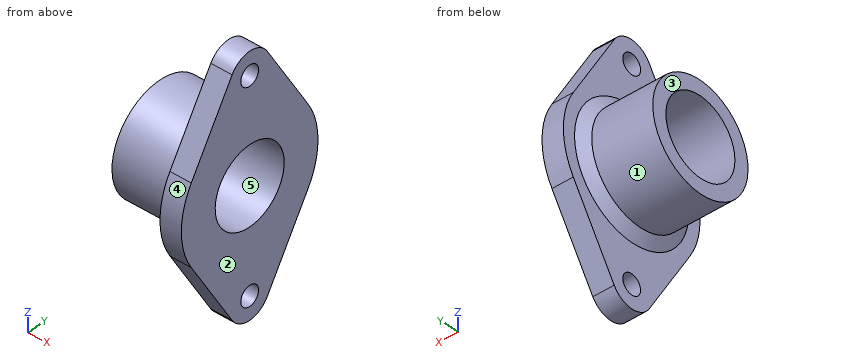
from build123d import *

# Parameters (mm, degrees)
BOSS_EXTRUDE1_DEPTH = 14
SKETCH2_R           = 6.5
CUT_EXTRUDE1_DEPTH  = 98.479485021
SKETCH3_R           = 25.25
CUT_EXTRUDE2_DEPTH  = 98.479485021
BOSS_EXTRUDE2_START = 45
SKETCH4_R           = 34.85
SKETCH4_R_2         = 25.25
BOSS_EXTRUDE2_DEPTH = 45


with BuildPart() as part:
    # Sketch1 → Boss-Extrude1 (new body)
    with BuildSketch(Plane(origin=(0, 0, 0), x_dir=(0, 0, -1), z_dir=(1, 0, 0))):
        with BuildLine():
            Line((-25.925925926, 42.753319928), (-75.277777778, 12.825995978))
            ThreePointArc((-75.277777778, 12.825995978), (-82.5, 0), (-75.277777778, -12.825995978))
            Line((-75.277777778, -12.825995978), (-25.925925926, -42.753319928))
            ThreePointArc((-25.925925926, -42.753319928), (0, -50), (25.925925926, -42.753319928))
            Line((25.925925926, -42.753319928), (75.277777778, -12.825995978))
            ThreePointArc((75.277777778, -12.825995978), (82.5, 0), (75.277777778, 12.825995978))
            Line((75.277777778, 12.825995978), (25.925925926, 42.753319928))
            ThreePointArc((25.925925926, 42.753319928), (0, 50), (-25.925925926, 42.753319928))
        make_face()
    extrude(amount=BOSS_EXTRUDE1_DEPTH)

    # Sketch2 → Cut-Extrude1 (cut, through all)
    with BuildSketch(Plane.ZY):
        with Locations((67.5, 0)):
            Circle(SKETCH2_R)
        with Locations((-67.5, 0)):
            Circle(SKETCH2_R)
    extrude(amount=-CUT_EXTRUDE1_DEPTH, mode=Mode.SUBTRACT)

    # Sketch3 → Cut-Extrude2 (cut, through all)
    with BuildSketch(Plane.ZY):
        Circle(SKETCH3_R)
    extrude(amount=-CUT_EXTRUDE2_DEPTH, mode=Mode.SUBTRACT)

    # Sketch4 → Boss-Extrude2 (add)
    with BuildSketch(Plane.ZY.offset(BOSS_EXTRUDE2_START)):
        with Locations(Location((0, 0, 0), (0, 0, 180))):
            Circle(SKETCH4_R)
        Circle(SKETCH4_R_2, mode=Mode.SUBTRACT)
    extrude(amount=-BOSS_EXTRUDE2_DEPTH)

    # Sketch5 → Revolve1 (revolve)
    with BuildSketch(Plane(origin=(0, 0, 0), x_dir=(1, 0, 0), z_dir=(0, 1, 0))):
        Polygon((0, 34.85), (-5, 34.85), (0, 41.85), align=None)
    revolve(axis=Axis((0, 0, 0), (-1, 0, 0)))


solid = part.part
Can you work these out from the model? Positions are in its coordinate system, mm. Face numbers are marked on the shaded views. A direction names the side the tool comes from. Coordinates: 2 decimals unless noted, no trailing zeros. Order: outer loops, then holes, each group sorted by start corner. A loop starts at its lowest first (then second) coordinate and runs counter-clockwise, first axis right, second up. Notation, with made-up numbers: M -21,-31.75 L -14,-31.75 A18 cw -14,-13.75 Z; hole C 80.5,21 d1. An arc over 180 degrees is marked long. Answer as CSV lines item,"result".
(1) If we mould it in two halves opening along Z, with no side actions, what happens to the marked faces 3, 4 and 5? For each: released by +Z, released by -Z, zero draft, split by the parting line, or undercut.
Geometry check:
face 3,"zero draft"
face 4,"split by the parting line"
face 5,"undercut"
(2) On a 3-axis mill with a long thin cutter (end or side, diameter ignored), from which of +Z, -Z, +X, -X, +Y, -Y can I reach the whole of each face in a straight line? I mean the marked faces 1 and 2. Say none if no direction works.
Geometry check:
face 1,"-X"
face 2,"+Z, -Z, +X, +Y, -Y"
(3) Suppose I cut it at C-C on x = -35. Please give me the cut outline in (y, z), plus the area to 3 significant figures.
Geometry check:
outline,"C 0,0 d69.7; hole C 0,0 d50.5"
area,"1,810 mm^2"
(4) I'm going to push flat-ended pins straight in: pin 1 (10.5 mm diameter, centred on y = 0, z = 67.5, fed in from -X); pin 2 (8 mm diameter, centred on x = 6.5, y = -29.5, fed in from +Z); pin 3 (2 mm diameter, centred on x = 5.5, z = -12, fed in from +Y) (3 decimals); pin 4 (10 mm diameter, centred on x = -8, z = 10, fed in from -Y). Where does each tip first touch, or does it pass through?
Geometry check:
pin 1,"through"
pin 2,"z = 54.38"
pin 3,"y = 48.775"
pin 4,"y = -36.42"
(5) Suppose I cut it at B-B on z = 0. Please give me the cut outline in (x, y), plus the area to 3 significant figures.
Geometry check:
outline,"M -45,-34.85 L -5,-34.85 L 0,-41.85 L 0,-50 L 14,-50 L 14,-25.25 L -45,-25.25 Z; M -45,25.25 L 14,25.25 L 14,50 L 0,50 L 0,41.85 L -5,34.85 L -45,34.85 Z"
area,"1,590 mm^2"
(6) Suppose I cut it at D-D on z = -67.5. Please give me the cut outline in (x, y).
Geometry check:
outline,"M 0,-17.54 L 14,-17.54 L 14,-6.5 L 0,-6.5 Z; M 0,6.5 L 14,6.5 L 14,17.54 L 0,17.54 Z"
(7) Suppose I cut it at A-A on y = 0. Please give me the cut outline in (x, z), plus the area to 3 significant figures.
Geometry check:
outline,"M -45,-34.85 L -5,-34.85 L 0,-41.85 L 0,-61 L 14,-61 L 14,-25.25 L -45,-25.25 Z; M -45,25.25 L 14,25.25 L 14,61 L 0,61 L 0,41.85 L -5,34.85 L -45,34.85 Z; M 0,-82.5 L 14,-82.5 L 14,-74 L 0,-74 Z; M 0,74 L 14,74 L 14,82.5 L 0,82.5 Z"
area,"2,140 mm^2"
(8) Please list where these lines run through material, in increasing order: L1, parallel to Y at x = -18.5, z = 0; L2, parallel to X at y = 20, z = 45; L3, parallel to Y at x = -28.5, z = -8.
Geometry check:
L1,"-34.85 to -25.25, 25.25 to 34.85"
L2,"0 to 14"
L3,"-33.92 to -23.95, 23.95 to 33.92"
